```python
from build123d import *

# Parameters (mm, degrees)
F0_R        = 4.5
F1_DEPTH    = 20
F2_W        = 7.0876832783
F2_H        = 5.546597673
F3_DEPTH    = 10
F4_DEPTH    = 12.5
F5_SIZE     = 1
F6_T4_ANGLE = 167.6048406122
F6_T9_ANGLE = 167.6048406122
F7_R        = 1


# Not quite as in the source:
# - a fillet or chamfer that OpenCascade refuses, or shapes differently, is made with other operations: its cross-section is extruded or revolved along the edge and cut away or added


with BuildPart() as f1:
    # F0 (on Top) → F1 (new body)
    with BuildSketch(Plane.XY):
        Circle(F0_R)
        with BuildLine():
            ThreePointArc((2.2, 1.1874342087), (2.4238399287, 0.6123724357), (2.5, 0))
            ThreePointArc((2.5, 0), (2.4238399287, -0.6123724357), (2.2, -1.1874342087))
            ThreePointArc((2.2, -1.1874342087), (-2.5, 0), (2.2, 1.1874342087))
        make_face(mode=Mode.SUBTRACT)
        with BuildLine():
            ThreePointArc((2.2, -1.1874342087), (2.4238399287, -0.6123724357), (2.5, 0))
            ThreePointArc((2.5, 0), (2.4238399287, 0.6123724357), (2.2, 1.1874342087))
            Line((2.2, 1.1874342087), (2.2, -1.1874342087))
        make_face()
    extrude(amount=F1_DEPTH)

    # F2 (on face) → F3 (join)
    with BuildSketch(Plane.XY.offset(20)):
        Rectangle(F2_W, F2_H)
        with BuildLine():
            Line((2.2, 1.1874342087), (2.2, -1.1874342087))
            ThreePointArc((2.2, -1.1874342087), (-2.5, 0), (2.2, 1.1874342087))
        make_face(mode=Mode.SUBTRACT)
    extrude(amount=F3_DEPTH)

    # F4 (add, symmetric): faces of the model
    f4_faces = [f1.faces().sort_by_distance(p)[0] for p in [
        (3.5438416392, 0, 25),
        (-3.5438416392, 0, 25),
    ]]
    extrude(f4_faces, amount=F4_DEPTH, both=True, dir=(1, 0, 0))

    # F5
    f5_edges = [f1.edges().sort_by_distance(p)[0] for p in [
        (0, -2.773299, 30),
        (0, 2.773299, 30),
        (16.043842, 0, 30),
        (-16.043842, 0, 30),
    ]]
    chamfer(f5_edges, length=F5_SIZE)

    # F6: fillet of radius 1 on 2 edges, made by hand


with BuildPart() as f6_tool2:
    # F6_s3 → F6_t4 (revolve)
    with BuildSketch(Plane(origin=(0, 0, 0), x_dir=(0, 0, 1), z_dir=(0.1079573604, -0.9941555252, 0))):
        with BuildLine():
            ThreePointArc((20, -3.5), (19.7071067812, -4.2071067812), (19, -4.5))
            Line((19, -4.5), (20, -4.5))
            Line((20, -4.5), (20, -3.5))
        make_face()
    revolve(axis=Axis((0, 0, 20), (0, 0, 1)), revolution_arc=F6_T4_ANGLE)

    split(bisect_by=Plane.XZ.offset(-2.7732988365), keep=Keep.BOTTOM)


with BuildPart() as f1_1:
    add(f1.part)

    # F6_t1: cut F6_tool2
    add(f6_tool2.part, mode=Mode.SUBTRACT)


with BuildPart() as f6_tool7:
    # F6_s8 → F6_t9 (revolve)
    with BuildSketch(Plane(origin=(0, 0, 0), x_dir=(0, 0, 1), z_dir=(-0.1079573604, 0.9941555252, 0))):
        with BuildLine():
            ThreePointArc((19, -4.5), (19.7071067812, -4.2071067812), (20, -3.5))
            Line((20, -3.5), (20, -4.5))
            Line((20, -4.5), (19, -4.5))
        make_face()
    revolve(axis=Axis((0, 0, 20), (0, 0, 1)), revolution_arc=F6_T9_ANGLE)

    split(bisect_by=Plane.XZ.offset(2.7732988365), keep=Keep.TOP)


with BuildPart() as f1_2:
    add(f1_1.part)

    # F6_t6: cut F6_tool7
    add(f6_tool7.part, mode=Mode.SUBTRACT)

    # F7
    f7_edges = [f1_2.edges().sort_by_distance(p)[0] for p in [
        (9.793842, 2.773299, 20),
        (-9.793842, 2.773299, 20),
        (9.793842, -2.773299, 20),
        (-9.793842, -2.773299, 20),
        (16.043842, 0, 20),
        (-16.043842, 0, 20),
    ]]
    fillet(f7_edges, radius=F7_R)


solid = f1_2.part
```
Can you work these out from the model? Positions are in its coordinate system, mm. A direction names the side the tool comes from. Give positions to 0.01 mm unless a question says otherwise; leave off trailing zeros. Loops run counter-clockwise (first coordinate to the right, second up) from the corner with the lowest first, then second, coordinate; pieces in that order, holes last. Notation, with made-up numbers: M 25,47 L 43,47 A22 ccw 43,72 Z; hole C -26,88 d4. An arc over 180 degrees is marked long. Answer in a Markdown table with one row per item.
1. If I drill on line 1 along Y through (x, z) = (0, 7); line 2 along X through (y, z) = (-1.75, 9.5); line 3 along Z through (x, y) = (9, 1.5), over which ranges is the centre line in solid material (lowest first)?
Taken from the geometry:
| item | result |
|---|---|
| line 1 | y = -4.5 to -2.5, 2.5 to 4.5 |
| line 2 | x = -4.15 to -1.79, 1.79 to 4.15 |
| line 3 | z = 20 to 30 |
2. Suppose I cut it at D-D on x = -7. Write out the boundary of the cut face in (y, z).
Taken from the geometry:
| item | result |
|---|---|
| outline | M -2.77,21 A1 ccw -1.77,20 L 1.77,20 A1 ccw 2.77,21 L 2.77,29 L 1.77,30 L -1.77,30 L -2.77,29 Z |
3. For pin 1 Ø1.8 at (x, y) = (-8.5, -0.5) entering from -Z; pin 2 Ø11 at (x, z) = (-6, 25.5) entering from -Y; pin 3 Ø1.2 at (y, z) = (0, 14.5) entering from -X, each with a flat end and sliding along its axis, tell me the tip position at first contact or that it passes through.
Taken from the geometry:
| item | result |
|---|---|
| pin 1 | stops at z = 20 |
| pin 2 | stops at y = -2.77 |
| pin 3 | stops at x = -4.5 |
4. Suppose I cut it at B-B on y = 0. Write out the boundary of the cut face in (x, z), plus the area to 3 significant figures.
Taken from the geometry:
| item | result |
|---|---|
| outline | M -16.04,21 A1 ccw -15.04,20 L -4.5,20 L -4.5,0 L -2.5,0 L -2.5,20 L 2.2,20 L 2.2,0 L 4.5,0 L 4.5,20 L 15.04,20 A1 ccw 16.04,21 L 16.04,29 L 15.04,30 L -15.04,30 L -16.04,29 Z |
| area | 405 mm² |
5. Thinking about a two-plate mould opening in Y: for faces 1 (the cylindrical face through (-9.706, 2.473, 20.285)), 2 (the flat face through (2, -2, 0)), 3 (the cylindrical face through (-2.5, -0.1, 9.9)), which applies, released by +Y, released by -Y, zero draft, split by the parting line, or undercut?
Taken from the geometry:
| item | result |
|---|---|
| face 1 | released by +Y |
| face 2 | zero draft |
| face 3 | undercut |
6. Which directions (+Z, -Z, +X, -X, +Y, -Y) give clear straight access to the entire face, cutting with the end or side of a thin tool? Please do faces 4 (the cylindrical face through (9.88, -2.49, 20.3)), 5 (the flat face through (2.2, 0, 10)), 6 (the cylindrical face through (9.881, 2.473, 20.285)), 7 (the cylindrical face through (-9.71, -2.49, 20.3)).
Taken from the geometry:
| item | result |
|---|---|
| face 4 | -Z, +X, -Y |
| face 5 | -Z |
| face 6 | -Z, +X, +Y |
| face 7 | -Z, -X, -Y |
7. Suppose I cut it at C-C on z = 14.5. Write out the boundary of the cut face in (x, y), plus the area to 3 significant figures.
Taken from the geometry:
| item | result |
|---|---|
| outline | C 0,0 d9; hole M 2.2,-1.19 L 2.2,1.19 A2.5 ccw long Z |
| area | 44.5 mm² |
8. Suppose I cut it at A-A on x = 0. Write out the boundary of the cut face in (y, z).
Taken from the geometry:
| item | result |
|---|---|
| outline | M -4.5,0 L -2.5,0 L -2.5,20 L 2.5,20 L 2.5,0 L 4.5,0 L 4.5,19 A1 ccw 3.5,20 L 2.77,20 L 2.77,29 L 1.77,30 L -1.77,30 L -2.77,29 L -2.77,20 L -3.5,20 A1 ccw -4.5,19 Z |
